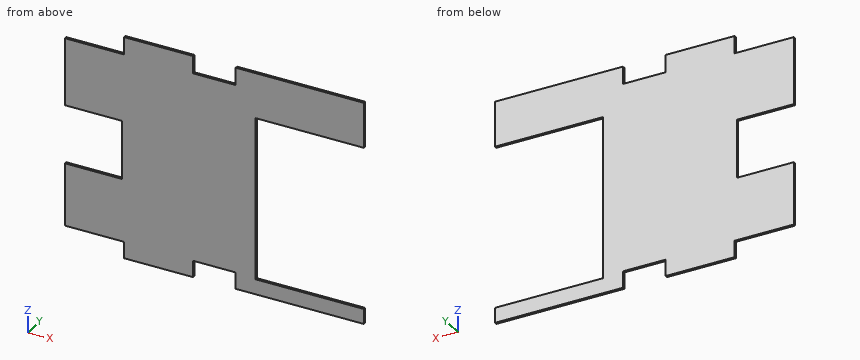
Autodesk Inventor part; units mm, degrees
ref_plane "YZ Plane" through (0, 0, 0) normal (1, 0, 0) x (0, 1, 0)
ref_plane "XZ Plane" through (0, 0, 0) normal (0, 1, 0) x (-1, 0, 0)
ref_plane "XY Plane" through (0, 0, 0) normal (0, 0, 1) x (1, 0, 0)
sketch "Sketch1" plane through (0, 0, 0) normal (0, 1, 0) x (-1, 0, 0)
  line L0 (234.95, 355.6) -> (-234.95, 355.6)
  line L1 (-234.95, 355.6) -> (-234.95, -355.6)
  line L2 (-234.95, -355.6) -> (234.95, -355.6)
  line L3 (234.95, -355.6) -> (234.95, 355.6)
  line L4 (234.95, 355.6) -> (-234.95, -355.6) construction
  line L5 (-234.95, 355.6) -> (234.95, -355.6) construction
  point P0 (0, 0)
  dimension "d0" = 469.9
  dimension "d1" = 711.2
extrude "Plate1" add sketch "Sketch1" along normal blind 3.048
sketch "Sketch3" plane through (0, 3.048, 0) normal (0, 1, 0) x (1, 0, 0)
  line L0 (234.95, -355.6) -> (-234.95, -355.6)
  point P0 (0, 0)
sketch "Sketch4" plane through (0, 0, 0) normal (0, -1, 0) x (1, 0, 0)
  line L0 (-234.95, 355.6) -> (234.95, 355.6)
  line L1 (-234.95, -355.6) -> (-234.95, 355.6)
  line L2 (234.95, -355.6) -> (-234.95, -355.6)
  line L3 (234.95, 355.6) -> (234.95, -355.6)
  line L4 (-234.95, 355.6) -> (234.95, 355.6)
  line L5 (25.4, 355.6) -> (25.4, 294.64)
  line L6 (165.1, 101.6) -> (234.95, 101.6)
  line L7 (234.95, 355.6) -> (234.95, -355.6)
  line L8 (25.4, 294.64) -> (165.1, 154.94)
  line L9 (25.4, 294.64) -> (222.9656, 294.64) construction
  line L10 (165.1, 154.94) -> (165.1, 101.6)
  line L11 (234.95, 0) -> (-234.95, 0)
  line L12 (-234.95, -355.6) -> (-234.95, 355.6)
  line L13 (25.4, -355.6) -> (25.4, -294.64)
  line L14 (165.1, -127) -> (234.95, -127)
  line L15 (25.4, -294.64) -> (165.1, -154.94)
  line L16 (25.4, -294.64) -> (222.9656, -294.64) construction
  line L17 (165.1, -154.94) -> (165.1, -127)
  line L18 (-234.95, 184.15) -> (-120.65, 184.15)
  line L19 (-120.65, 184.15) -> (-120.65, 177.8)
  line L20 (-120.65, 177.8) -> (-222.25, 177.8)
  line L21 (-222.25, 177.8) -> (-222.25, 152.4)
  line L22 (-222.25, 152.4) -> (-234.95, 152.4)
  line L23 (-234.95, 149.86) -> (-219.71, 149.86)
  line L24 (-219.71, 149.86) -> (-219.71, 175.26)
  line L25 (-219.71, 175.26) -> (-118.11, 175.26)
  line L26 (-118.11, 175.26) -> (-118.11, 186.69)
  line L27 (-118.11, 186.69) -> (-234.95, 186.69)
  line L28 (165.1, -129.54) -> (20.32, -129.54)
  line L29 (20.32, -129.54) -> (20.32, 88.9)
  line L30 (20.32, 88.9) -> (165.1, 88.9)
  line L31 (165.1, 101.6) -> (165.1, 88.9)
  line L32 (-234.95, -184.15) -> (-120.65, -184.15)
  line L33 (-120.65, -184.15) -> (-120.65, -177.8)
  line L34 (-120.65, -177.8) -> (-222.25, -177.8)
  line L35 (-222.25, -177.8) -> (-222.25, -152.4)
  line L36 (-222.25, -152.4) -> (-234.95, -152.4)
  line L37 (-234.95, -149.86) -> (-219.71, -149.86)
  line L38 (-219.71, -149.86) -> (-219.71, -175.26)
  line L39 (-219.71, -175.26) -> (-118.11, -175.26)
  line L40 (-118.11, -175.26) -> (-118.11, -186.69)
  line L41 (-118.11, -186.69) -> (-234.95, -186.69)
  line L42 (-158.75, 35.56) -> (-158.75, -43.18)
  line L43 (-158.75, -43.18) -> (-234.95, -43.18)
  line L44 (-158.75, 35.56) -> (-234.95, 35.56)
  line L45 (25.4, 330.2) -> (6.35, 330.2)
  line L46 (6.35, 330.2) -> (6.35, 355.6)
  line L47 (25.4, -330.2) -> (6.35, -330.2)
  line L48 (6.35, -330.2) -> (6.35, -355.6)
  line L49 (234.95, -355.6) -> (-234.95, -355.6)
  point P0 (0, 0)
  dimension "d3" = 209.55
  dimension "d4" = 254
  dimension "d5" = 45
  dimension "d6" = 60.96
  dimension "d9" = 69.85
  dimension "d12" = 45
  dimension "d13" = 209.55
  dimension "d14" = 228.6
  dimension "d15" = 69.85
  dimension "d16" = 60.96
  dimension "d17" = 171.45
  dimension "d18" = 114.3
  dimension "d19" = 6.35
  dimension "d21" = 101.6
  dimension "d22" = 25.4
  dimension "d23" = 2.54
  dimension "d26" = 144.78
  dimension "d31" = 12.7
  dimension "d32" = 114.3
  dimension "d33" = 171.45
  dimension "d34" = 6.35
  dimension "d35" = 101.6
  dimension "d36" = 25.4
  dimension "d37" = 2.54
  dimension "d38" = 76.2
  dimension "d39" = 35.56
  dimension "d40" = 43.18
  dimension "d41" = 2.54
  dimension "d42" = 25.4
  dimension "d43" = 19.05
  dimension "d44" = 25.4
  dimension "d45" = 19.05
extrude "Cut1" cut sketch "Sketch4" against normal blind 3.048 contours L27 L26 L25 L24 L23 L1 L22 L21 L20 L19 L18 | L0 L3 L6 L10 L8 L5 | L18 L19 L20 L21 L22 L1 | L3 L11 L29 L30 L31 L6 | L3 L14 L17 L28 L29 L11 | L44 L42 L11 L1 | L3 L2 L13 L15 L17 L14 | L11 L42 L43 L1 | L37 L38 L39 L40 L41 L1 L32 L33 L34 L35 L36 | L36 L35 L34 L33 L32 L1
sketch "Sketch5" plane through (0, 0, 0) normal (0, -1, 0) x (1, 0, 0)
  line L0 (25.4, 355.6) -> (25.4, 294.64)
  line L1 (25.4, 294.64) -> (165.1, 154.94)
  line L2 (165.1, 154.94) -> (165.1, 88.9)
  line L3 (165.1, 88.9) -> (20.32, 88.9)
  line L4 (20.32, 88.9) -> (20.32, -129.54)
  line L5 (20.32, -129.54) -> (165.1, -129.54)
  line L6 (165.1, -129.54) -> (165.1, -154.94)
  line L7 (165.1, -154.94) -> (25.4, -294.64)
  line L8 (25.4, -294.64) -> (25.4, -355.6)
  line L9 (25.4, -355.6) -> (-234.95, -355.6)
  line L10 (-234.95, -355.6) -> (-234.95, -186.69)
  line L11 (-234.95, -186.69) -> (-118.11, -186.69)
  line L12 (-118.11, -186.69) -> (-118.11, -175.26)
  line L13 (-118.11, -175.26) -> (-219.71, -175.26)
  line L14 (-219.71, -175.26) -> (-219.71, -149.86)
  line L15 (-219.71, -149.86) -> (-234.95, -149.86)
  line L16 (-234.95, -149.86) -> (-234.95, -43.18)
  line L17 (-234.95, -43.18) -> (-158.75, -43.18)
  line L18 (-158.75, -43.18) -> (-158.75, 35.56)
  line L19 (-158.75, 35.56) -> (-234.95, 35.56)
  line L20 (-234.95, 35.56) -> (-234.95, 149.86)
  line L21 (-234.95, 149.86) -> (-219.71, 149.86)
  line L22 (-219.71, 149.86) -> (-219.71, 175.26)
  line L23 (-219.71, 175.26) -> (-118.11, 175.26)
  line L24 (-118.11, 175.26) -> (-118.11, 186.69)
  line L25 (-118.11, 186.69) -> (-234.95, 186.69)
  line L26 (-234.95, 186.69) -> (-234.95, 355.6)
  line L27 (-234.95, 355.6) -> (25.4, 355.6)
  line L28 (25.4, -355.6) -> (-234.95, -355.6)
  line L29 (25.4, -355.6) -> (6.35, -355.6)
  line L30 (6.35, -355.6) -> (6.35, -330.2)
  line L31 (6.35, -330.2) -> (25.4, -330.2)
  line L32 (25.4, -330.2) -> (25.4, -355.6)
  line L33 (-234.95, 355.6) -> (25.4, 355.6)
  line L34 (25.4, 355.6) -> (6.35, 355.6)
  line L35 (6.35, 355.6) -> (6.35, 330.2)
  line L36 (6.35, 330.2) -> (25.4, 330.2)
  line L37 (25.4, 330.2) -> (25.4, 355.6)
  line L38 (-146.05, -355.6) -> (-101.6, -355.6)
  line L39 (-101.6, -355.6) -> (-101.6, -330.2)
  line L40 (-101.6, -330.2) -> (-146.05, -330.2)
  line L41 (-146.05, -330.2) -> (-146.05, -355.6)
  line L42 (-146.05, 355.6) -> (-101.6, 355.6)
  line L43 (-101.6, 355.6) -> (-101.6, 330.2)
  line L44 (-101.6, 330.2) -> (-146.05, 330.2)
  line L45 (-146.05, 330.2) -> (-146.05, 355.6)
  point P0 (0, 0)
  dimension "d46" = 19.05
  dimension "d47" = 25.4
  dimension "d48" = 19.05
  dimension "d49" = 25.4
  dimension "d52" = 44.45
  dimension "d53" = 25.4
  dimension "d54" = 88.9
  dimension "d55" = 44.45
  dimension "d56" = 25.4
  dimension "d57" = 88.9
extrude "Cut2" cut sketch "Sketch5" against normal blind 3.048 contours L0 L36 L35 L27 | L43 L44 L45 L27 | L8 L9 L30 L31 | L9 L41 L40 L39
sketch "Sketch6" plane through (0, 3.048, 0) normal (0, 1, 0) x (1, 0, 0)
  line L0 (20.32, -88.9) -> (165.1, -88.9)
  line L1 (165.1, -88.9) -> (165.1, -154.94)
  line L2 (165.1, -154.94) -> (25.4, -294.64)
  line L3 (25.4, -294.64) -> (25.4, -330.2)
  line L4 (25.4, -330.2) -> (6.35, -330.2)
  line L5 (6.35, -330.2) -> (6.35, -355.6)
  line L6 (6.35, -355.6) -> (-101.6, -355.6)
  line L7 (-101.6, -355.6) -> (-101.6, -330.2)
  line L8 (-101.6, -330.2) -> (-146.05, -330.2)
  line L9 (-146.05, -330.2) -> (-146.05, -355.6)
  line L10 (-146.05, -355.6) -> (-234.95, -355.6)
  line L11 (-234.95, -355.6) -> (-234.95, -186.69)
  line L12 (-234.95, -186.69) -> (-118.11, -186.69)
  line L13 (-118.11, -186.69) -> (-118.11, -175.26)
  line L14 (-118.11, -175.26) -> (-219.71, -175.26)
  line L15 (-219.71, -175.26) -> (-219.71, -149.86)
  line L16 (-219.71, -149.86) -> (-234.95, -149.86)
  line L17 (-234.95, -149.86) -> (-234.95, -35.56)
  line L18 (-234.95, -35.56) -> (-158.75, -35.56)
  line L19 (-158.75, -35.56) -> (-158.75, 43.18)
  line L20 (-158.75, 43.18) -> (-234.95, 43.18)
  line L21 (-234.95, 43.18) -> (-234.95, 149.86)
  line L22 (-234.95, 149.86) -> (-219.71, 149.86)
  line L23 (-219.71, 149.86) -> (-219.71, 175.26)
  line L24 (-219.71, 175.26) -> (-118.11, 175.26)
  line L25 (-118.11, 175.26) -> (-118.11, 186.69)
  line L26 (-118.11, 186.69) -> (-234.95, 186.69)
  line L27 (-234.95, 186.69) -> (-234.95, 355.6)
  line L28 (-234.95, 355.6) -> (-146.05, 355.6)
  line L29 (-146.05, 355.6) -> (-146.05, 330.2)
  line L30 (-146.05, 330.2) -> (-101.6, 330.2)
  line L31 (-101.6, 330.2) -> (-101.6, 355.6)
  line L32 (-101.6, 355.6) -> (6.35, 355.6)
  line L33 (6.35, 355.6) -> (6.35, 330.2)
  line L34 (6.35, 330.2) -> (25.4, 330.2)
  line L35 (25.4, 330.2) -> (25.4, 294.64)
  line L36 (25.4, 294.64) -> (165.1, 154.94)
  line L37 (165.1, 154.94) -> (165.1, 129.54)
  line L38 (165.1, 129.54) -> (20.32, 129.54)
  line L39 (20.32, 129.54) -> (20.32, -88.9)
  line L40 (-234.95, -151.765) -> (-155.575, -151.765)
  line L41 (-155.575, -151.765) -> (-155.575, -126.365)
  line L42 (-155.575, -126.365) -> (-234.95, -126.365)
  line L43 (-234.95, -126.365) -> (-234.95, -151.765)
  line L44 (-234.95, -151.765) -> (-155.575, -126.365) construction
  line L45 (-155.575, -151.765) -> (-234.95, -126.365) construction
  line L46 (85.725, -151.765) -> (165.1, -151.765)
  line L47 (165.1, -151.765) -> (165.1, -126.365)
  line L48 (165.1, -126.365) -> (85.725, -126.365)
  line L49 (85.725, -126.365) -> (85.725, -151.765)
  line L50 (85.725, -151.765) -> (165.1, -126.365) construction
  line L51 (165.1, -151.765) -> (85.725, -126.365) construction
  line L52 (165.1, -154.94) -> (165.1, -88.9)
  line L53 (-234.95, -149.86) -> (-234.95, -35.56)
  line L54 (85.725, 127.635) -> (165.1, 127.635)
  line L55 (165.1, 127.635) -> (165.1, 153.035)
  line L56 (165.1, 153.035) -> (85.725, 153.035)
  line L57 (85.725, 153.035) -> (85.725, 127.635)
  line L58 (85.725, 127.635) -> (165.1, 153.035) construction
  line L59 (165.1, 127.635) -> (85.725, 153.035) construction
  line L60 (-63.5, 127.635) -> (-6.35, 127.635)
  line L61 (-6.35, 127.635) -> (-6.35, 153.035)
  line L62 (-6.35, 153.035) -> (-63.5, 153.035)
  line L63 (-63.5, 153.035) -> (-63.5, 127.635)
  line L64 (-63.5, 127.635) -> (-6.35, 153.035) construction
  line L65 (-6.35, 127.635) -> (-63.5, 153.035) construction
  line L66 (-63.5, -151.765) -> (-6.35, -151.765)
  line L67 (-6.35, -151.765) -> (-6.35, -126.365)
  line L68 (-6.35, -126.365) -> (-63.5, -126.365)
  line L69 (-63.5, -126.365) -> (-63.5, -151.765)
  line L70 (-63.5, -151.765) -> (-6.35, -126.365) construction
  line L71 (-6.35, -151.765) -> (-63.5, -126.365) construction
  line L72 (-195.2625, -139.065) -> (125.4125, -139.065) construction
  line L73 (-234.95, 127.635) -> (-155.575, 127.635)
  line L74 (-155.575, 127.635) -> (-155.575, 153.035)
  line L75 (-155.575, 153.035) -> (-234.95, 153.035)
  line L76 (-234.95, 153.035) -> (-234.95, 127.635)
  line L77 (-234.95, 127.635) -> (-155.575, 153.035) construction
  line L78 (-155.575, 127.635) -> (-234.95, 153.035) construction
  line L79 (-155.575, -151.765) -> (85.725, -151.765)
  line L80 (85.725, 153.035) -> (-155.575, 153.035)
  line L81 (-234.95, -35.56) -> (-234.95, -149.86) construction
  line L82 (-234.95, -149.86) -> (165.1, -149.86)
  line L83 (-234.95, 149.86) -> (165.1, 149.86)
  line L84 (165.1, 154.94) -> (165.1, 129.54) construction
  point P0 (0, 0)
  point P1 (125.4125, 140.335)
  point P2 (-34.925, 140.335)
  point P3 (-34.925, -139.065)
  point P4 (-34.925, -139.065)
  point P5 (-195.2625, 140.335)
  point P6 (-63.5, 153.035)
  point P7 (-6.35, 153.035)
  point P8 (-6.35, -151.765)
  point P9 (-63.5, -151.765)
  point P10 (-63.5, -149.86)
  point P11 (-155.575, -149.86)
  point P12 (-6.35, -149.86)
  point P13 (165.1, -149.86)
  point P14 (-6.35, 149.86)
  point P15 (-155.575, 149.86)
  point P16 (-63.5, 149.86)
  dimension "d58" = 25.4
  dimension "d59" = 3.175
  dimension "d60" = 79.375
  dimension "d61" = 57.15
  dimension "d62" = 279.4
extrude "Extrusion1" cut sketch "Sketch6" against normal through all contours L1 L46 L49 L82 | L83 L61 L80 L57 | L57 L56 L37 L83 | L1 L2 L3 L4 L5 L6 L7 L8 L9 L10 L11 L12 L13 L14 L15 L40 L79 L66 L46 | L49 L79 L67 L82 | L80 L62 L75 L23 L24 L25 L26 L27 L28 L29 L30 L31 L32 L33 L34 L35 L36 L37 L56 | L83 L63 L62 L61 | L61 L60 L63 L83 | L82 L69 L68 L67 | L67 L66 L69 L82 | L83 L74 L80 L63 | L69 L79 L41 L82 | L83 L23 L75 L74 | L74 L73 L21 L22 L83 | L82 L16 L17 L42 L41 | L41 L40 L15 L82
equation "\"d10\" = Thickness"
equation "\"d2\" = Thickness"
equation "\"BendRadius\" = Thickness"
equation "\"BendReliefWidth\" = Thickness"
equation "\"BendReliefDepth\" = 0.5 * Thickness"
equation "\"CornerReliefSize\" = 4 * Thickness"
equation "\"MinimumRemnant\" = 2 * Thickness"
equation "\"TransitionRadius\" = BendRadius"
equation "\"JacobiRadiusSize\" = BendRadius"
equation "\"GapSize\" = Thickness"
properties part number "DB1-020" material "Polycarbonate, Smoke"
Can you work these out from the model? Positions are in its coordinate system, mm. Give positions to 0.01 mm unless a question says otherwise; leave off trailing zeros. Loops run counter-clockwise (first coordinate to the right, second up) from the corner with the lowest first, then second, coordinate; pieces in that order, holes last. Notation, with made-up numbers: M -36,83 L -14,83 A15 ccw -14,96 Z; hole C 38,-3.75 d11. An arc over 180 degrees is marked long. One line per question, with ' | ' between items. Start each with the question number.
Q1. If we section it at B-B (y = 1.5): Please give me the cut outline in (x, z) (3 decimals).
Q2. If we section it at C-C (z = 27): Please give me the cut outline in (x, y), plus the area to 3 significant figures.
Q3. If I drill on line 1 (Z direction, x = 44, y = 0.85); line 2 (X direction, y = 1, z = 130) (3 decimals); line 3 (Z direction, x = -196.5, y = 0.8) (3 decimals), over which ranges is the centre line in solid material (lowest first)? Write a range as from..to.
Q4. For pin 1 Ø1.5 at (y, z) = (1, 135.5) entering from -X (3 decimals); pin 2 Ø1.5 at (y, z) = (2, 8) entering from -X; pin 3 Ø0.9 at (x, y) = (-197, 1) entering from +Z (3 decimals), each with a flat end and sliding along its axis, tell me the tip position at first contact or that it passes through.
Q5. If we section it at A-A (x = 97.5): Please give me the cut outline in (y, z), plus the area to 3 significant figures.
Computed:
1) outline: M -234.95,-127.635 L -155.575,-127.635 L -155.575,-149.86 L -63.5,-149.86 L -63.5,-127.635 L -6.35,-127.635 L -6.35,-149.86 L 165.1,-149.86 L 165.1,-129.54 L 20.32,-129.54 L 20.32,88.9 L 165.1,88.9 L 165.1,149.86 L -6.35,149.86 L -6.35,126.365 L -63.5,126.365 L -63.5,149.86 L -155.575,149.86 L -155.575,126.365 L -234.95,126.365 L -234.95,35.56 L -158.75,35.56 L -158.75,-43.18 L -234.95,-43.18 Z
2) outline: M -158.75,0 L 20.32,0 L 20.32,3.05 L -158.75,3.05 Z | area: 546 mm²
3) line 1: z = -149.86..-129.54, 88.9..149.86 | line 2: x = -155.575..-63.5, -6.35..165.1 | line 3: z = -127.635..-43.18, 35.56..126.365
4) pin 1: stops at x = -155.575 | pin 2: stops at x = -158.75 | pin 3: stops at z = 126.365
5) outline: M 0,-149.86 L 3.05,-149.86 L 3.05,-129.54 L 0,-129.54 Z; M 0,88.9 L 3.05,88.9 L 3.05,149.86 L 0,149.86 Z | area: 248 mm²
